Source: three-view drawing plus pictorial views. Frame: mm from the lowest corner of the part. Give positions to 0.01 mm unless a question says otherwise; leave off trailing zeros. Order: outer loops, then holes, each group sorted by start corner. A loop starts at its lowest first (then second) coordinate and runs counter-clockwise, first axis right, second up.
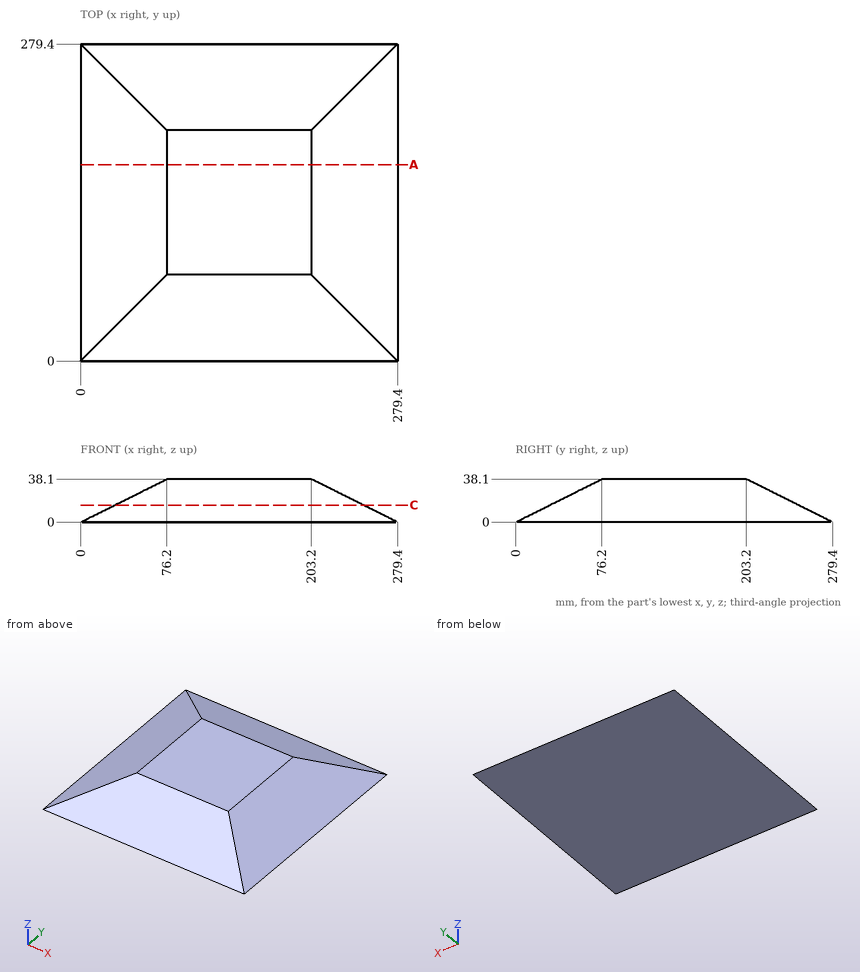
1) Section query C-C on z = 15. Output: boundary loops of the cut face in (x, y).
Checks:
outline: (30, 30) - (249.4, 30) - (249.4, 249.4) - (30, 249.4) - close
2) First-contact query: pin 1 Ø1.5 at (y, z) = (151.5, 11.5) entering from +X; pin 2 Ø1 at (x, z) = (225.5, 14) entering from +Y; pin 3 Ø3 at (x, y) = (231, 63.5) entering from +Z. Flat tips, straight axial feed; report the tip coordinate or a pass-through.
Checks:
pin 1: stops at x = 257.9
pin 2: stops at y = 252.4
pin 3: stops at z = 24.95
3) Section query A-A on y = 173. Output: boundary loops of the cut face in (x, z).
Checks:
outline: (0, 0) - (279.4, 0) - (203.2, 38.1) - (76.2, 38.1) - close
4) Ray query, L1, parallel to Z at x = 57, y = 175; L2, parallel to Y at x = 193.5, z = 35; L3, parallel to Z at x = 31, y = 112. Return the intervals inside material, ascending.
Checks:
L1: z = 0 to 28.5
L2: y = 70 to 209.4
L3: z = 0 to 15.5
